Geometry check sheet. Reference: the model listing, model coordinates, mm. A direction names the side the tool comes from. Round coordinates to 2 decimals unless told otherwise and drop trailing zeros. Loops run counter-clockwise (first coordinate to the right, second up) from the corner with the lowest first, then second, coordinate; pieces in that order, holes last. Notation, with made-up numbers: M -38,-28 L 20,-28 A20 cw 20,-17 Z; hole C -26,55.5 d4. An arc over 180 degrees is marked long. Answer in a Markdown table with one row per item. Add a question column.
```python
from build123d import *
from build123d.topology import SkipClean

# Parameters (mm, degrees)
SKETCH1_R                 = 82
SKETCH1_R_2               = 50
BOSS_EXTRUDE1_DEPTH       = 1
BOSS_EXTRUDE3_START       = 11
SKETCH3_R                 = 82
SKETCH3_R_2               = 75
BOSS_EXTRUDE3_DEPTH       = 11
SKETCH4_R                 = 5
CUT_EXTRUDE1_DEPTH        = 117.584733134
CIRPATTERN1_COUNT         = 4
CUT_EXTRUDE3_DEPTH        = 11
CIRPATTERN3_COUNT         = 4
M2X0_4_TAPPED_HOLE1_D     = 1.6
M2X0_4_TAPPED_HOLE1_DEPTH = 10
M2X0_4_TAPPED_HOLE1_TIP   = 0.480688495


with BuildPart() as part:
    # Sketch1 → Boss-Extrude1 (new body)
    with BuildSketch(Plane.XY):
        Circle(SKETCH1_R)
        Circle(SKETCH1_R_2, mode=Mode.SUBTRACT)
    extrude(amount=BOSS_EXTRUDE1_DEPTH)

    # Sketch3 → Boss-Extrude3 (add)
    with BuildSketch(Plane(origin=(0, 0, 0), x_dir=(-1, 0, 0), z_dir=(0, 0, -1)).offset(BOSS_EXTRUDE3_START)):
        Circle(SKETCH3_R)
        Circle(SKETCH3_R_2, mode=Mode.SUBTRACT)
    extrude(amount=-BOSS_EXTRUDE3_DEPTH)

    # Sketch4 → Cut-Extrude1 (cut, through all)
    with SkipClean():  # the faces are left unmerged after this step: merging them gives an invalid solid
        with BuildSketch(Plane.XY.offset(1)):
            with Locations((0, 83)):
                Circle(SKETCH4_R)
        cut_extrude1 = extrude(amount=-CUT_EXTRUDE1_DEPTH, mode=Mode.SUBTRACT)

    # CirPattern1: Cut-Extrude1 ×4 about axis
    cirpattern1_axis = Axis((0, 0, 0), (0, 0, 1))
    for i in range(1, CIRPATTERN1_COUNT):
        add(cut_extrude1.rotate(cirpattern1_axis, i * 360 / CIRPATTERN1_COUNT), mode=Mode.SUBTRACT)

    # Sketch6 → Cut-Extrude3 (cut)
    with BuildSketch(Plane(origin=(0, 0, -11), x_dir=(-1, 0, 0), z_dir=(0, 0, -1))):
        Polygon((38.066313572, 46.551594946), (59.467914625, 67.953195999), (67.882250994, 59.39696962), (46.551594946, 38.066313572), align=None)
    cut_extrude3 = extrude(amount=-CUT_EXTRUDE3_DEPTH, mode=Mode.SUBTRACT)

    # CirPattern3: Cut-Extrude3 ×4 about axis
    cirpattern3_axis = Axis((0, 0, 0), (0, 0, 1))
    for i in range(1, CIRPATTERN3_COUNT):
        add(cut_extrude3.rotate(cirpattern3_axis, i * 360 / CIRPATTERN3_COUNT), mode=Mode.SUBTRACT)

    # M2x0.4 Tapped Hole1
    with Locations(Plane(origin=(41.000000001, 71.01408311, -5), x_dir=(0.86602540378, -0.500000000007, 0), z_dir=(0.500000000007, 0.86602540378, 0))):
        with Locations((0, 0)):
            Hole(M2X0_4_TAPPED_HOLE1_D / 2, depth=M2X0_4_TAPPED_HOLE1_DEPTH)
            with Locations((0, 0, -(M2X0_4_TAPPED_HOLE1_DEPTH + M2X0_4_TAPPED_HOLE1_TIP / 2))):  # 118° drill point
                Cone(0, M2X0_4_TAPPED_HOLE1_D / 2, M2X0_4_TAPPED_HOLE1_TIP, mode=Mode.SUBTRACT)


solid = part.part
```
1) Cross-section at A-A, the plane z = -9. Record the boundary of the cut face in (x, y), plus the area to 3 significant figures.
2) Set-up check for faces 1 (the flat face through (-51.068, 59.553, -5.577)), 2 (the flat face through (-59.553, -51.068, -5.577)), 3 (the flat face through (59.553, 51.068, -5.577)): record each of +Z, -Z, +X, -X, +Y, -Y from which the full face is reachable in a straight line by a thin tool's end or side.
3) Go/stop test with flat-tipped pins: pin 1 (4 mm diameter, centred on y = 27, z = -4.5, fed in from -X); pin 2 (3 mm diameter, centred on y = -22, z = -1.5, fed in from -X); pin 3 (6 mm diameter, centred on x = -39, z = -3, fed in from +Y); pin 4 (12 mm diameter, centred on x = 32, y = -25.5, fed in from +Z). Record where each tip stops, or that it passes through.
4) Cross-section at B-B, the plane x = 0. Record the boundary of the cut face in (y, z).
5) Thickness scan on L1, parallel to Z at x = 29, y = 64.5; L2, parallel to X at y = -16.5, z = -0.75; L3, parallel to X at y = 23, z = -1.5. Record the ranges inside material, lowest first. Write a range as [from, to].
6) Draft check along X on faces 4 (the cylindrical face through (0, 78, -5)), 5 (the flat face through (51.068, -59.553, -5.577)), 6 (the flat face through (-76, -4, -11)). Enter one of: +X half, -X half, draft (parallel to the pull), parting line (faces both ways), or undercut.
Worked answers:
| question | item | result |
|---|---|---|
| 1 | outline | M -81.86,-4.87 A82 ccw -62.07,-53.58 L -57.11,-48.62 A75 cw -57.11,48.62 L -62.07,53.58 A82 ccw -81.86,4.87 A5 cw Z; M -53.58,-62.07 A82 ccw -4.87,-81.86 A5 cw 4.87,-81.86 A82 ccw 53.58,-62.07 L 48.62,-57.11 A75 cw -48.62,-57.11 Z; M -53.58,62.07 L -48.62,57.11 A75 cw 48.62,57.11 L 53.58,62.07 A82 ccw 4.87,81.86 A5 cw -4.87,81.86 A82 ccw Z; M 57.11,-48.62 L 62.07,-53.58 A82 ccw 81.86,-4.87 A5 cw 81.86,4.87 A82 ccw 62.07,53.58 L 57.11,48.62 A75 cw Z |
| 1 | area | 3,000 mm2 |
| 2 | face 1 | -Z, -X |
| 2 | face 2 | -Z, -Y |
| 2 | face 3 | -Z, +Y |
| 3 | pin 1 | stops at x = -78.1 |
| 3 | pin 2 | stops at x = -79.4 |
| 3 | pin 3 | stops at y = 73.67 |
| 3 | pin 4 | passes through |
| 4 | outline | M -78,-11 L -75,-11 L -75,0 L -50,0 L -50,1 L -78,1 Z; M 50,0 L 75,0 L 75,-11 L 78,-11 L 78,1 L 50,1 Z |
| 5 | L1 | z = [0, 1] |
| 5 | L2 | x = [-80.32, -73.16], [73.16, 80.32] |
| 5 | L3 | x = [-78.71, -71.39], [71.39, 78.71] |
| 6 | face 4 | undercut |
| 6 | face 5 | +X half |
| 6 | face 6 | draft |
